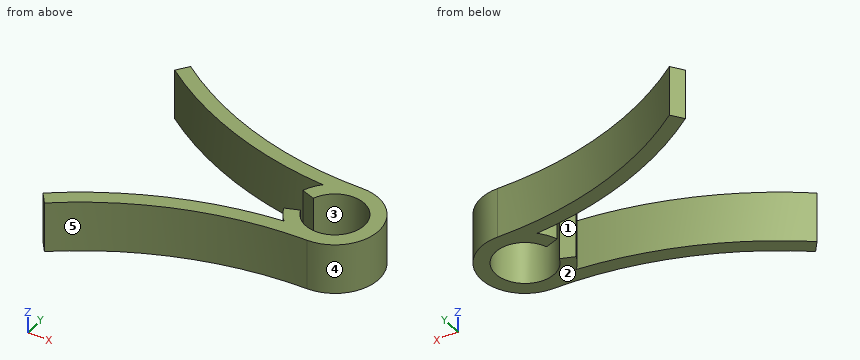
Autodesk Inventor part; units mm, degrees
ref_plane "YZ Plane" through (0, 0, 0) normal (1, 0, 0) x (0, 1, 0)
ref_plane "XZ Plane" through (0, 0, 0) normal (0, 1, 0) x (-1, 0, 0)
ref_plane "XY Plane" through (0, 0, 0) normal (0, 0, 1) x (1, 0, 0)
sketch "Sketch1" plane through (0, 0, 0) normal (0, 0, 1) x (1, 0, 0)
  circle A0 centre (0, 0) radius 4.1
  circle A1 centre (0, 0) radius 6.1
  arc A2 (-30, 16.1) -> (0, 6.1) centre (0, 56.1) ccw
  line L0 (0, -78.54) -> (0, 78.54)
  arc A3 (-31.2, 14.5) -> (0, 4.1) centre (0, 56.1) ccw
  line L1 (-30, 16.1) -> (-31.2, 14.5)
  line L2 (-39.6726, 0) -> (13.7288, 0)
  arc A4 (0, -6.1) -> (-30, -16.1) centre (0, -56.1) ccw
  arc A5 (0, -4.1) -> (-31.2, -14.5) centre (0, -56.1) ccw
  line L3 (-30, -16.1) -> (-31.2, -14.5)
  line L4 (-5.7321, 2.0863) -> (-3.8527, 1.4023)
  line L5 (-5.7321, -2.0863) -> (-3.8527, -1.4023)
  point P0 (0, 4.1)
  point P1 (0, -4.1)
  point P2 (0, -6.1)
  point P3 (-3.8527, -1.4023)
  point P4 (-4.3447, -4.2818)
  point P5 (-4.3447, 4.2818)
  dimension "d0" = 8.2
  dimension "d1" = 2
  dimension "d3" = 50
  dimension "d4" = 30
  dimension "d7" = 20
extrude "Extrusion1" add sketch "Sketch1" along normal blind 7 contours L2 A1 L0 A0 | A0 L0 A1 L2 | A3 A1 L0 | A0 L4 A1 A3 | A5 A1 L5 A0 | L0 A1 A5 | A1 A3 L1 A2 | A4 L3 A5 A1
properties part number "8mmClamp"
CAD build for the part. Positions are in the model's coordinates, mm. Face numbers are marked on the shaded views. A direction names the side the tool comes from. Coordinates: 2 decimals unless noted, no trailing zeros. Order: outer loops, then holes, each group sorted by start corner. A loop starts at its lowest first (then second) coordinate and runs counter-clockwise, first axis right, second up. Notation, with made-up numbers: (49.25, 87.25) - (78.25, 87.25) arc R34 ccw to (78.25, 123.25) - close; hole circle Ø10 at (87.5, 55.5). An arc over 180 degrees is marked (long way). Use a Markdown table: item, result. Add a question column.
(1) Drill centre lines: line 1 along Y through (x, z) = (0, 4.75); line 2 along X through (y, z) = (0, 2.5); line 3 along Y through (x, z) = (-5, 5). Where is each one in solid material? Low to high. Write a range as [from, to].
(2) Saw through at B-B (y = 0). Give the cut face in (x, z).
(3) Flat gauge pins, fed straight in: pin 1 (3 mm diameter, centred on y = 5.5, z = 5, fed in from +X); pin 2 (1 mm diameter, centred on y = 10, z = 6, fed in from -X); pin 3 (3 mm diameter, centred on y = 12, z = 4.5, fed in from -X). Where does each tip first touch, or does it go through?
(4) Saw through at C-C (z = 1). Give the cut face in (x, y).
(5) Pull direction Y, two halves, no side cores. Call the marked faces 3, 4 and 5: +Y half, -Y half, draft (parallel to the pull), parting line (faces both ways), or undercut.
(6) Saw through at A-A (x = -17). Give the cut face in (y, z).
(7) Which spindle directions (+Z, -Z, +X, -X, +Y, -Y) get a long thin tool onto all of the face, cutting with end or side? Do the marked faces 1 and 2. Say none if no direction does.
(8) Saw through at D-D (y = -8.5). Give the cut face in (x, z), then the cut area to 3 significant figures.
Solved:
| question | item | result |
|---|---|---|
| 1 | line 1 | y = [-6.1, -4.1], [4.1, 6.1] |
| 1 | line 2 | x = [4.1, 6.1] |
| 1 | line 3 | y = [-6.35, -4.34], [-3.49, -1.82], [1.82, 3.49], [4.34, 6.35] |
| 2 | outline | (4.1, 0) - (6.1, 0) - (6.1, 7) - (4.1, 7) - close |
| 3 | pin 1 | stops at x = 4.61 |
| 3 | pin 2 | stops at x = -24.99 |
| 3 | pin 3 | stops at x = -29.82 |
| 4 | outline | (-31.2, -14.5) - (-30, -16.1) arc R50 cw to (0, -6.1) arc R6.1 ccw to (0, 6.1) arc R50 cw to (-30, 16.1) - (-31.2, 14.5) arc R52 ccw to (-4.34, 4.28) arc R6.1 ccw to (-5.73, 2.09) - (-3.85, 1.4) arc R4.1 cw (long way) to (-3.85, -1.4) - (-5.73, -2.09) arc R6.1 ccw to (-4.34, -4.28) arc R52 ccw to start |
| 5 | face 3 | undercut |
| 5 | face 4 | parting line |
| 5 | face 5 | -Y half |
| 6 | outline | (-9.08, 0) - (-6.96, 0) - (-6.96, 7) - (-9.08, 7) - close; (6.96, 0) - (9.08, 0) - (9.08, 7) - (6.96, 7) - close |
| 7 | face 1 | +Z, -Z, -X |
| 7 | face 2 | -Z, +X, -X, +Y, -Y |
| 8 | outline | (-20.93, 0) - (-15.3, 0) - (-15.3, 7) - (-20.93, 7) - close |
| 8 | area | 39.4 mm² |
